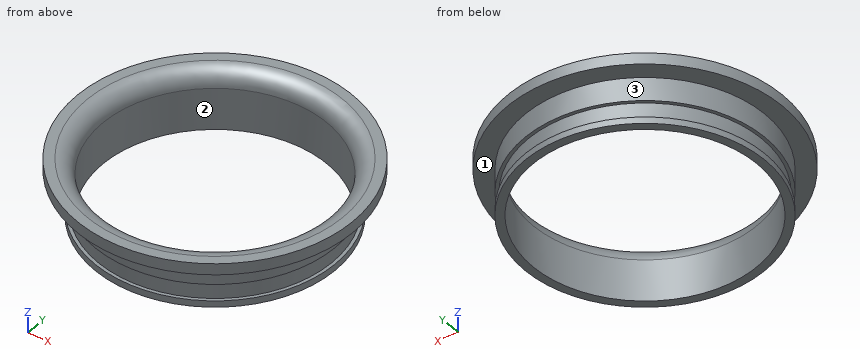
from build123d import *

# Parameters (mm, degrees)
F0_R     = 37.5
F0_R_2   = 35
F1_DEPTH = 18
F2_R     = 43
F2_R_2   = 35
F3_DEPTH = 3.5
F4_R     = 5
F6_R     = 37.5
F6_R_2   = 36.5
F7_DEPTH = 5.2


with BuildPart() as f1:
    # F0 (on Top) → F1 (new body)
    with BuildSketch(Plane.XY):
        Circle(F0_R)
        Circle(F0_R_2, mode=Mode.SUBTRACT)
    extrude(amount=F1_DEPTH)

    # F2 (on face) → F3 (join)
    with BuildSketch(Plane.XY.offset(18)):
        Circle(F2_R)
        Circle(F2_R_2, mode=Mode.SUBTRACT)
    extrude(amount=-F3_DEPTH)

    # F4
    f4_edges = [f1.edges().sort_by_distance(p)[0] for p in [
        (-35, 0, 18),
    ]]
    fillet(f4_edges, radius=F4_R)

    # F6 (on offset) → F7 (cut)
    with BuildSketch(Plane(origin=(0, 0, 2), x_dir=(1, 0, 0), z_dir=(0, 0, -1))):
        Circle(F6_R)
        Circle(F6_R_2, mode=Mode.SUBTRACT)
    extrude(amount=-F7_DEPTH, mode=Mode.SUBTRACT)


solid = f1.part
Model file for the job. Use its own axes, mm. Face numbers are marked on the shaded views. Give positions to 0.01 mm unless a question says otherwise; leave off trailing zeros. Write each loop counter-clockwise with the first axis right and the second up, starting at its lowest first coordinate (ties: lowest second). Pieces come first, ordered by that corner, then holes. Notation, with made-up numbers: (24.5, 74.25) -> (42.5, 74.25) arc R22 cw to (42.5, 108.25) -> close; hole circle Ø5 at (-15, -13.5). An arc over 180 degrees is marked (long way). Write item = value, one per line.
(1) Slice it at D-D, the plane z = 10. Give the cut face in (x, y).
Determined:
outline = circle Ø75 at (0, 0); hole circle Ø70 at (0, 0)
(2) Mould opens along X. For the marked faces 1, 2 and 3 say: released by +X, released by -X, zero draft, split by the parting line, or undercut.
Determined:
face_1 = zero draft
face_2 = undercut
face_3 = split by the parting line
(3) Flat gauge pins, fed straight in: P1, Ø6, axis at y = 12, z = 8.5, coming from the -X side; P2, Ø22.5, axis at x = 17, y = 7, coming from the -Z side (3 decimals); P3, Ø1.5, axis at y = 22, z = 12, coming from the -X side; P4, Ø12, axis at x = 31.5, y = 10, coming from the +Z side. Where does each tip first touch, or does it go through?
Determined:
P1 = -36.4
P2 = through
P3 = -30.9
P4 = 17.91
(4) Slice it at A-A, the plane y = 0. Give the cut face in (x, z), then the cut area to 3 significant figures.
Determined:
outline = (-43, 14.5) -> (-37.5, 14.5) -> (-37.5, 7.2) -> (-36.5, 7.2) -> (-36.5, 2) -> (-37.5, 2) -> (-37.5, 0) -> (-35, 0) -> (-35, 13) arc R5 ccw to (-40, 18) -> (-43, 18) -> close; (35, 0) -> (37.5, 0) -> (37.5, 2) -> (36.5, 2) -> (36.5, 7.2) -> (37.5, 7.2) -> (37.5, 14.5) -> (43, 14.5) -> (43, 18) -> (40, 18) arc R5 ccw to (35, 13) -> close
area = 107 mm2
(5) Probe line 1 along Y through (x, z) = (0, 5.75); line 2 along Y through (x, z) = (0, 9.5); line 3 along X through (y, z) = (11.5, 8.5). List the from-to ranges inside material, lowest first.
Determined:
line_1 = -36.5 to -35, 35 to 36.5
line_2 = -37.5 to -35, 35 to 37.5
line_3 = -35.69 to -33.06, 33.06 to 35.69
(6) Slice it at C-C, the plane z = 4.5. Give the cut face in (x, y), then the cut area to 3 significant figures.
Determined:
outline = circle Ø73 at (0, 0); hole circle Ø70 at (0, 0)
area = 337 mm2
